Autodesk Inventor part; units mm, degrees
ref_plane "YZ Plane" through (0, 0, 0) normal (1, 0, 0) x (0, 1, 0)
ref_plane "XZ Plane" through (0, 0, 0) normal (0, 1, 0) x (-1, 0, 0)
ref_plane "XY Plane" through (0, 0, 0) normal (0, 0, 1) x (1, 0, 0)
sketch "Sketch1" plane through (0, 0, 0) normal (1, 0, 0) x (0, 1, 0)
  line L0 (0, 0) -> (533.4, 0)
  line L1 (533.4, 0) -> (533.4, -508)
  line L2 (533.4, -508) -> (0, -508)
  line L3 (0, -508) -> (0, 0)
  dimension "d0" = 533.4
  dimension "d1" = 508
extrude "Extrusion1" add sketch "Sketch1" along normal blind 1.5875
sketch "Sketch3" plane through (0, 0, 0) normal (-1, 0, 0) x (0, 0, 1)
  line L0 (-508, 0) -> (-508, 533.4)
  line L1 (0, 0) -> (-508, 0)
  circle A0 centre (-358.14, 12.7) radius 3.302
  circle A1 centre (-358.14, 25.4) radius 3.302
  circle A2 centre (-149.86, 12.7) radius 3.302
  circle A3 centre (-149.86, 25.4) radius 3.302
  circle A4 centre (-254, 12.7) radius 3.302
  circle A5 centre (-254, 25.4) radius 3.302
  circle A6 centre (-358.14, 508) radius 3.302
  circle A7 centre (-358.14, 520.7) radius 3.302
  circle A8 centre (-149.86, 508) radius 3.302
  circle A9 centre (-149.86, 520.7) radius 3.302
  circle A10 centre (-254, 508) radius 3.302
  circle A11 centre (-254, 520.7) radius 3.302
extrude "Extrusion5" cut sketch "Sketch3" against normal up to surface (1.5875 mm away) contours A0 | A1 | A2 | A3 | A4 | A5
sheet face with bend "Face1" sketch "Sketch1" thickness 3.048 toward (1, 0, 0) bend radius 3.048
bend "Bend1"
extrude "Cut1" cut sketch "Sketch3" against normal up to surface (3.048 mm away)
sketch "Sketch4" plane through (3.048, 0, 0) normal (1, 0, 0) x (0, 0, -1)
  line L0 (508, 533.4) -> (508, 0)
  line L1 (508, 266.7) -> (434.34, 266.7)
  line L2 (0, 0) -> (508, 0)
  line L3 (434.34, 0) -> (434.34, 34.925)
  line L4 (434.34, 0) -> (469.265, 0) construction
  line L5 (434.34, 34.925) -> (349.377, 34.925)
  line L6 (434.34, 17.4625) -> (346.202, 17.4625)
  line L7 (346.202, 0) -> (346.202, 31.75)
  line L8 (346.202, 31.75) -> (349.377, 34.925)
  line L9 (434.34, 533.4) -> (434.34, 498.475)
  line L10 (434.34, 498.475) -> (349.377, 498.475)
  line L11 (434.34, 515.9375) -> (346.202, 515.9375)
  line L12 (346.202, 533.4) -> (346.202, 501.65)
  line L13 (346.202, 501.65) -> (349.377, 498.475)
  line L14 (0, 533.4) -> (508, 533.4)
  line L15 (508, 0) -> (0, 0)
  dimension "d42" = 73.66
  dimension "d43" = 34.925
  dimension "d44" = 90
  dimension "d45" = 84.963
  dimension "d46" = 88.138
  dimension "d47" = 31.75
extrude "Cut2" cut sketch "Sketch4" against normal blind 3.048
equation "\"d38\" = Thickness"
equation "\"d48\" = Thickness"
equation "\"d32\" = Thickness"
equation "\"d33\" = BendRadius"
equation "\"d34\" = BendReliefWidth"
equation "\"d36\" = MinimumRemnant"
equation "\"d35\" = BendReliefDepth"
equation "\"d37\" = TransitionRadius"
equation "\"BendRadius\" = Thickness"
equation "\"BendReliefWidth\" = Thickness"
equation "\"BendReliefDepth\" = 0.5 * Thickness"
equation "\"CornerReliefSize\" = 4 * Thickness"
equation "\"MinimumRemnant\" = 2 * Thickness"
equation "\"TransitionRadius\" = BendRadius"
equation "\"JacobiRadiusSize\" = BendRadius"
equation "\"GapSize\" = Thickness"
properties part number "TopV5" material "Acrylic, Clear"
Work out the finished part from the listing and answer in its coordinate system (mm). Round coordinates to 2 decimals unless told otherwise and drop trailing zeros. Loops run counter-clockwise (first coordinate to the right, second up) from the corner with the lowest first, then second, coordinate; pieces in that order, holes last. Notation, with made-up numbers: (72, -39.5) - (102, -39.5) arc R17 ccw to (102, -31.5) - close; hole circle Ø2 at (-3, 0). An arc over 180 degrees is marked (long way). Use one line per item in the form item = value. Start each with the question number.
(1) Find section B-B on z = -388.5. Determine the outline of the cut face in (x, y) (3 decimals), and give its area (3 significant figures).
(2) Find section A-A on x = 1.9. Give the number of separate pieces and of enclosed holes in the cut face, and give its area (3 significant figures).
(3) Flat-ended cylindrical pins translate along their axes: P1, Ø7.5, axis at y = 25.4, z = -149.86, coming from the +X side; P2, Ø0.9, axis at x = 1, z = -413, coming from the +Y side (3 decimals). Find the tip coordinate at first contact, or state that the pin passes through.
(4) Consider line 1 (Z direction, x = 2, y = 520.7); line 2 (Y direction, x = 1.2, z = -149.86). Determine where each line is inside the solid, lowest interval first.
Answer list:
q1.outline = (0, 34.925) - (3.048, 34.925) - (3.048, 498.475) - (0, 498.475) - close
q1.area = 1,410 mm^2
q2.separate_pieces = 1
q2.enclosed_holes = 8
q2.area = 265,000 mm^2
q3.P1 = 3.05
q3.P2 = 498.475
q4.line_1 = -508 to -434.34, -346.2 to -257.3, -250.7 to -153.16, -146.56 to 0
q4.line_2 = 0 to 9.4, 16 to 22.1, 28.7 to 504.7, 511.3 to 517.4, 524 to 533.4
